Geometry: see drawing. Coordinates: mm, zero at the bounding-box minimum. A direction names the side the tool comes from. Coordinates: 2 decimals unless noted, no trailing zeros. Write each loop counter-clockwise with the first axis right and the second up, starting at its lowest first coordinate (ties: lowest second). Pieces come first, ordered by that corner, then holes. Notation, with made-up numbers: (21, 27.5) -> (58, 27.5) arc R22 cw to (58, 34.5) -> close; hole circle Ø8 at (-33, 80.5). An arc over 180 degrees is marked (long way). Answer as a JSON object with one key per item and string values. Group by question number.
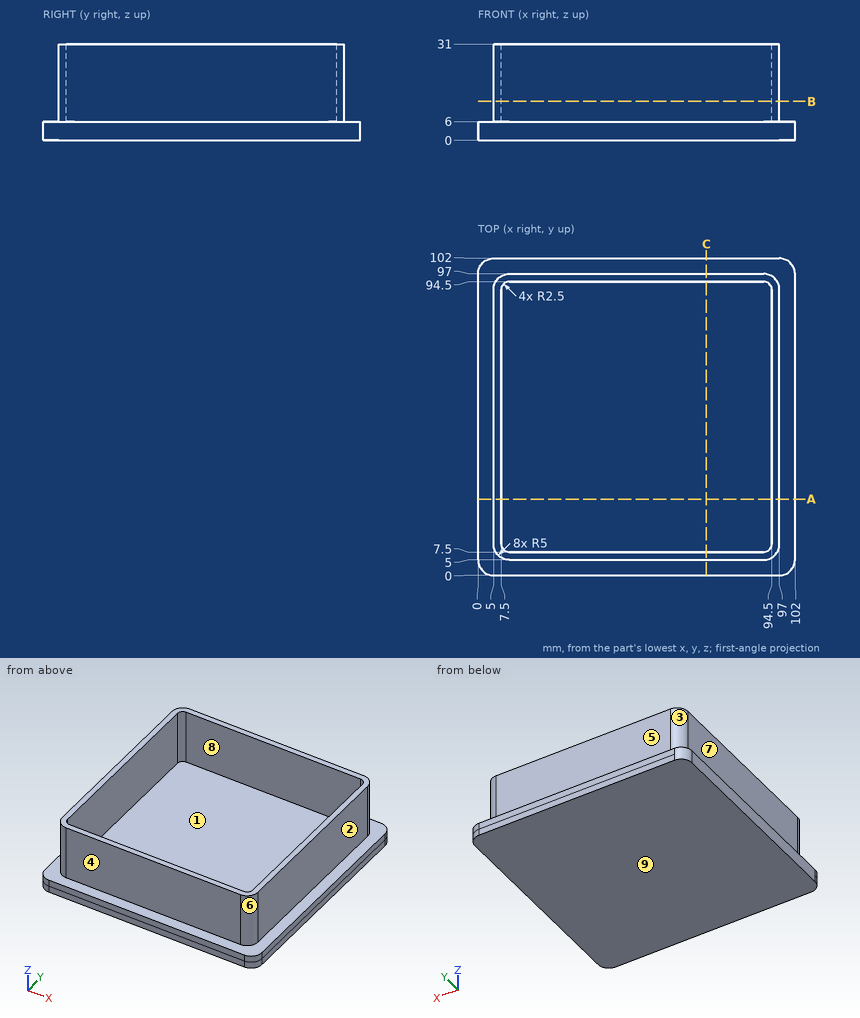
Item 1: Contact query for flat-ended pins moving along their axis: pin 1 (12.5 mm diameter, centred on y = 55, z = 22, fed in from +X); pin 2 (12 mm diameter, centred on x = 25, y = 16, fed in from +Z); pin 3 (2 mm diameter, centred on x = 59, z = 22.5, fed in from +Y). Output: stop coordinate, or through.
Item 2: Section B-B on z = 12.5. Output: boundary loops of the cut face in (x, y), then the cut area to 3 significant figures.
Item 3: Section A-A on y = 24.5. Output: boundary loops of the cut face in (x, z).
Item 4: Mould query, pull axis X, two halves, no side actions, for the marked faces 6, 7, 8 and 9. Classes: +X half, -X half, draft (parallel to the pull), parting line (faces both ways), or undercut.
Item 5: Set-up query: the marked faces 1, 2, 3, 4 and 5. Return all of +Z, -Z, +X, -X, +Y, -Y with unobstructed straight access to the full face (end or side cutting, diameter ignored); none if empty.
Item 6: Ray query, L1, parallel to X at y = 86.5, z = 22; L2, parallel to Z at x = 53.5, y = 13.5. Return the intervals inside material, ascending. Write a range as [from, to].
Answer sheet:
{
 "1": {"pin 1": "stops at x = 97", "pin 2": "stops at z = 6", "pin 3": "stops at y = 97"},
 "2": {"outline": "(5, 10) arc R5 ccw to (10, 5) -> (92, 5) arc R5 ccw to (97, 10) -> (97, 92) arc R5 ccw to (92, 97) -> (10, 97) arc R5 ccw to (5, 92) -> close; hole (7.5, 10) arc R2.5 ccw to (10, 7.5) -> (92, 7.5) arc R2.5 ccw to (94.5, 10) -> (94.5, 92) arc R2.5 ccw to (92, 94.5) -> (10, 94.5) arc R2.5 ccw to (7.5, 92) -> close", "area": "879 mm^2"},
 "3": {"outline": "(0, 0) -> (102, 0) -> (102, 6) -> (97, 6) -> (97, 31) -> (94.5, 31) -> (94.5, 6) -> (7.5, 6) -> (7.5, 31) -> (5, 31) -> (5, 6) -> (0, 6) -> close"},
 "4": {"face 6": "+X half", "face 7": "-X half", "face 8": "undercut", "face 9": "draft"},
 "5": {"face 1": "+Z", "face 2": "+Z, +X, +Y, -Y", "face 3": "+Z, -X, +Y", "face 4": "+Z, +X, -X, -Y", "face 5": "+Z, +X, -X, +Y"},
 "6": {"L1": "x = [5, 7.5], [94.5, 97]", "L2": "z = [0, 6]"}
}
